Check sheet for the drawn part. Datum: minimum x, y, z corner. Units: mm. Coordinates: 2 decimals unless noted, no trailing zeros. Write each loop counter-clockwise with the first axis right and the second up, starting at its lowest first coordinate (ties: lowest second). Pieces come first, ordered by that corner, then holes. Notation, with made-up numbers: (13, -9.75) - (38, -9.75) arc R18 ccw to (38, 23.25) - close; hole circle Ø3 at (34, 66). An arc over 180 degrees is marked (long way). Answer as CSV lines item,"result". Start each with the question number.
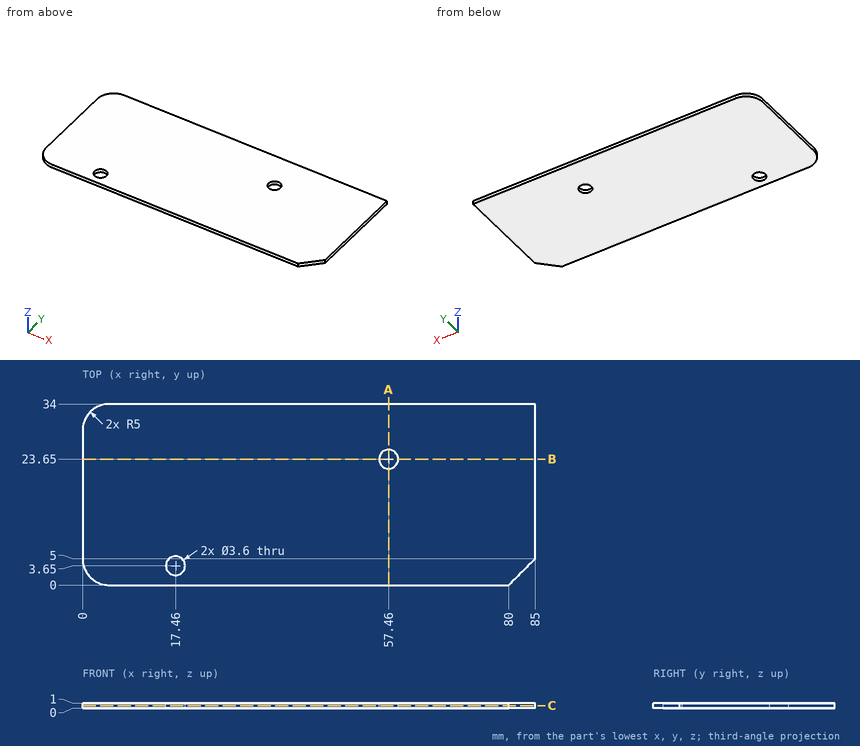
(1) Cross-section at B-B on y = 23.65. Record the boundary of the cut face in (x, z), plus the area to 3 significant figures.
(2) Cross-section at C-C on z = 0.55. Record the boundary of the cut face in (x, y), plus the area to 3 significant figures.
(3) Material ranges on probe 1 along Y at (x, z) = (17.46, 0.45); probe 2 along Y at (x, z) = (57.46, 0.35); probe 3 along X at (y, z) = (30, 0.7), recorded low to high. Write a range as from..to.
(4) Cross-section at A-A on x = 57.46. Record the boundary of the cut face in (y, z), plus the area to 3 significant figures.
(5) Go/stop test with a flat-tipped pin: P1, Ø3, axis at x = 57.46, y = 23.65, coming from the -Z side. Record where the tip stops, or that it passes through.
Checked values:
1,outline,"(0, 0) - (55.66, 0) - (55.66, 1) - (0, 1) - close; (59.26, 0) - (85, 0) - (85, 1) - (59.26, 1) - close"
1,area,"81.4 mm^2"
2,outline,"(0, 5) arc R5 ccw to (5, 0) - (80, 0) - (85, 5) - (85, 34) - (5, 34) arc R5 ccw to (0, 29) - close; hole circle Ø3.6 at (17.46, 3.65); hole circle Ø3.6 at (57.46, 23.65)"
2,area,"2,850 mm^2"
3,probe 1,"0..1.85, 5.45..34"
3,probe 2,"0..21.85, 25.45..34"
3,probe 3,"0.1..85"
4,outline,"(0, 0) - (21.85, 0) - (21.85, 1) - (0, 1) - close; (25.45, 0) - (34, 0) - (34, 1) - (25.45, 1) - close"
4,area,"30.4 mm^2"
5,P1,"through"
